Autodesk Inventor part; units mm, degrees
ref_plane "YZ Plane" through (0, 0, 0) normal (1, 0, 0) x (0, 1, 0)
ref_plane "XZ Plane" through (0, 0, 0) normal (0, 1, 0) x (-1, 0, 0)
ref_plane "XY Plane" through (0, 0, 0) normal (0, 0, 1) x (1, 0, 0)
sketch "Sketch1" plane through (0, 0, 0) normal (0, 1, 0) x (-1, 0, 0)
  line L0 (-10.5, 20) -> (10.5, 20)
  line L1 (10.5, 20) -> (10.5, -20)
  line L2 (10.5, -20) -> (-10.5, -20)
  line L3 (-10.5, -20) -> (-10.5, 20)
  line L4 (-10.5, 20) -> (10.5, -20) construction
  line L5 (10.5, 20) -> (-10.5, -20) construction
  point P0 (0, 0)
  dimension "d0" = 40
  dimension "d1" = 21
extrude "Extrusion1" add sketch "Sketch1" along normal blind 2
sketch "Sketch2" plane through (0, 2, 0) normal (0, 1, 0) x (1, 0, 0)
  line L0 (-10.5, 20) -> (-10.5, -20)
  line L1 (-10.5, -20) -> (10.5, -20)
  line L2 (10.5, -20) -> (10.5, 20)
  line L3 (10.5, 20) -> (-10.5, 20)
  point P0 (0, 0)
  point P1 (-9, -18.5)
  point P2 (-9, 18.5)
  point P3 (9, 18.5)
  point P4 (9, -18.5)
  dimension "d4" = 1.5
  dimension "d5" = 1.5
  dimension "d6" = 1.5
  dimension "d7" = 1.5
  dimension "d20" = 18
  dimension "d21" = 18
  dimension "d22" = 37
hole "Hole1" at (-9, 2, 18.5) at (-9, 2, -18.5) at (9, 2, -18.5) at (9, 2, 18.5) direction (0, -1, 0) diameter 2.2 end through all
sketch "Sketch3" plane through (0, 2, 0) normal (0, 1, 0) x (1, 0, 0)
  line L0 (7.5, -13.5) -> (-6.5, -13.5)
  line L1 (-6.5, -13.5) -> (-6.5, 16.5)
  line L2 (-6.5, 16.5) -> (7.5, 16.5)
  line L3 (7.5, 16.5) -> (7.5, -13.5)
  line L4 (7.5, -13.5) -> (-6.5, 16.5) construction
  line L5 (-6.5, -13.5) -> (7.5, 16.5) construction
  line L6 (-10.5, -20) -> (10.5, -20)
  line L7 (-10.5, 20) -> (-10.5, -20)
  line L8 (10.5, 20) -> (-10.5, 20)
  point P0 (0, 0)
  point P1 (0.5, 1.5)
  point P2 (0, -20)
  dimension "d15" = 6.5
  dimension "d16" = 30
  dimension "d17" = 14
  dimension "d18" = 4
  dimension "d19" = 3.5
extrude "Extrusion2" add sketch "Sketch3" along normal blind 7
properties part number "7_Seg_Display_TM1637"
The model under review builds one solid part; all positions refer to its coordinate system, in mm. A direction names the side the tool comes from. Coordinates: 2 decimals unless noted, no trailing zeros. Write each loop counter-clockwise with the first axis right and the second up, starting at its lowest first coordinate (ties: lowest second). Pieces come first, ordered by that corner, then holes. Notation, with made-up numbers: (55, -3.5) - (99, -3.5) arc R27 ccw to (99, 32.5) - close; hole circle Ø2 at (-27, -7). An arc over 180 degrees is marked (long way). Answer in a Markdown table with one row per item. Add a question column.
Q1. For faces 5 (the face through (1, 5, 13.5)), 6 (the face through (-6.5, 5, -1)), 7 (the face through (7.5, 5, -2)), list the 3-axis set-ups (+Z, -Z, +X, -X, +Y, -Y) from which the entire face can be reached by the end or side of a thin tool; tool diameter is ignored.
Q2. Draft analysis for pull direction Z (two halves, no side actions). For faces 1 (the face through (0, 1, -20)), 2 (the face through (9, 1, -19.6)), 3 (the face through (-7, 2, 0)), 4 (the face through (-9, 1, -19.6)), state which applies: +Z half, -Z half, draft (parallel to the pull), parting line (faces both ways), or undercut.
Q3. Consider section A-A on z = 18.5. Give the boundary of the cut face in (x, y).
Q4. Consider section C-C on x = -4.5. Give the boundary of the cut face in (y, z), then the cut area to 3 significant figures.
Q5. Clearance check with flat-ended pins moving along their axes: pin 1 (2.5 mm diameter, centred on x = -9, z = -18.5, fed in from +Y); pin 2 (3 mm diameter, centred on x = 2, y = 8, fed in from -Z); pin 3 (1.5 mm diameter, centred on x = 5, y = 6, fed in from +Z); pin 4 (1.3 mm diameter, centred on x = 9, z = -18.5, fed in from +Y). State where each tip first meets the part, or that it passes through.
Q6. Consider section B-B on x = -9. Give the boundary of the cut face in (y, z), then the cut area to 3 significant figures.
Q7. To check wall thickness, follow line 1 along X through (y, z) = (0.85, -18.5); line 2 along Z through (x, y) = (-9, 1); line 3 along Y through (x, z) = (8.5, 0.5). State the ranges of each line that lie inside material, in increasing order. Write a range as from..to.
Q8. Consider section D-D on z = -5.5. Give the boundary of the cut face in (x, y).
Answers below:
| question | item | result |
|---|---|---|
| 1 | face 5 | +Z, +X, -X, +Y |
| 1 | face 6 | +Z, -Z, -X, +Y |
| 1 | face 7 | +Z, -Z, +X, +Y |
| 2 | face 1 | -Z half |
| 2 | face 2 | undercut |
| 2 | face 3 | draft |
| 2 | face 4 | undercut |
| 3 | outline | (-10.5, 0) - (-10.1, 0) - (-10.1, 2) - (-10.5, 2) - close; (-7.9, 0) - (7.9, 0) - (7.9, 2) - (-7.9, 2) - close; (10.1, 0) - (10.5, 0) - (10.5, 2) - (10.1, 2) - close |
| 4 | outline | (0, -20) - (2, -20) - (2, -16.5) - (9, -16.5) - (9, 13.5) - (2, 13.5) - (2, 20) - (0, 20) - close |
| 4 | area | 290 mm² |
| 5 | pin 1 | y = 2 |
| 5 | pin 2 | z = -16.5 |
| 5 | pin 3 | z = 13.5 |
| 5 | pin 4 | through |
| 6 | outline | (0, -20) - (2, -20) - (2, -19.6) - (0, -19.6) - close; (0, -17.4) - (2, -17.4) - (2, 17.4) - (0, 17.4) - close; (0, 19.6) - (2, 19.6) - (2, 20) - (0, 20) - close |
| 6 | area | 71.2 mm² |
| 7 | line 1 | -10.5..-10.1, -7.9..7.9, 10.1..10.5 |
| 7 | line 2 | -20..-19.6, -17.4..17.4, 19.6..20 |
| 7 | line 3 | 0..2 |
| 8 | outline | (-10.5, 0) - (10.5, 0) - (10.5, 2) - (7.5, 2) - (7.5, 9) - (-6.5, 9) - (-6.5, 2) - (-10.5, 2) - close |
